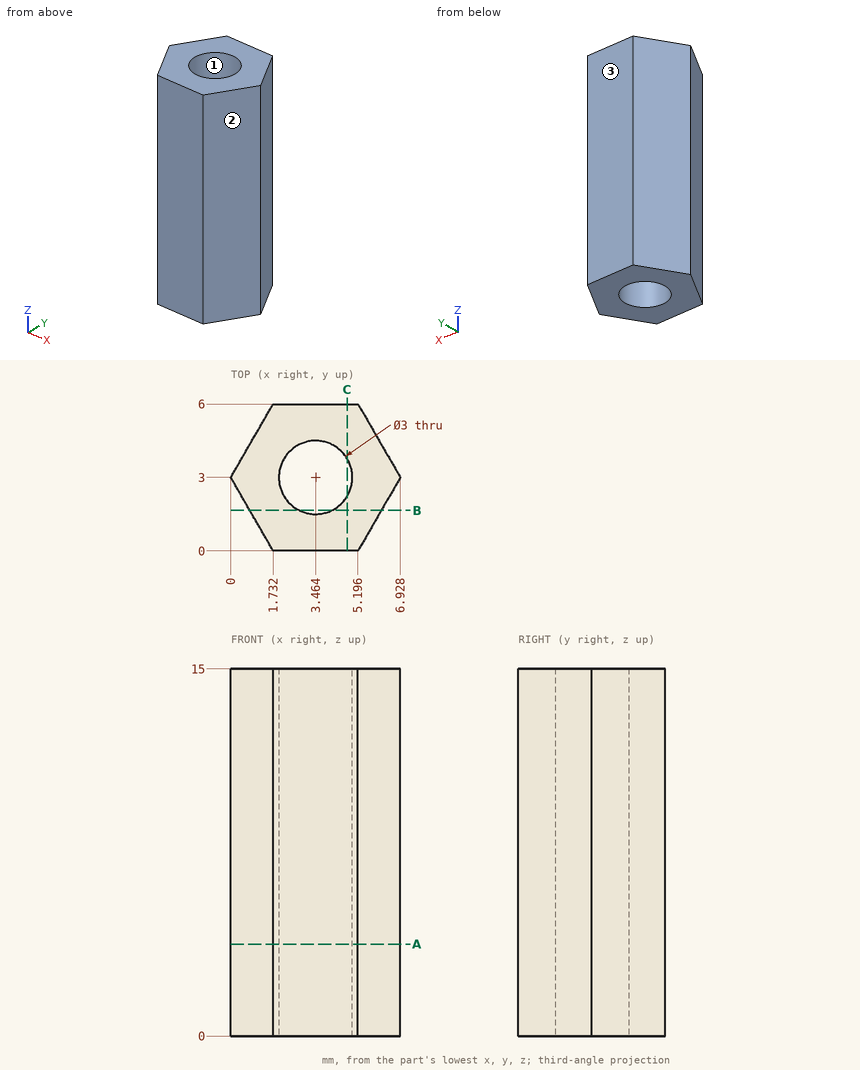
For this review, use the dimensioned drawing (mm, ordinates from the lowest corner) and the shaded views. Coordinates: 2 decimals unless noted, no trailing zeros. Order: outer loops, then holes, each group sorted by start corner. A loop starts at its lowest first (then second) coordinate and runs counter-clockwise, first axis right, second up. Notation, with made-up numbers: (-3, 63) -> (41, 63) arc R19 ccw to (41, 70) -> close; hole circle Ø1 at (52.5, 30.25). An arc over 180 degrees is marked (long way). One line per item, written item: value. Start each with the question number.
Q1. Take a section at A-A, the plane z = 3.75. State the section outline as (x, y) points.
Q2. Mouldability with a two-part tool opening along Y and no side actions: class the marked faces 1, 2 and 3 as pulls with the +Y half, pulls with the -Y half, needs draft (parallel to the pull), parting line crosses it, or undercut.
Q3. Take a section at C-C, the plane x = 4.75. State the section outline as (y, z) points.
Q4. Take a section at B-B, the plane y = 1.65. State the section outline as (x, z) points.
Q5. Insertion check: pin 1 Ø3 at (y, z) = (2, 5.5) entering from +X. The pin has a flat end and moves straight along its axis. Give the tip position at first contact, or say it passes through.
Q6. For probe 1 along X at (y, z) = (2.25, 13) (1 decimal); probe 2 along Y at (x, z) = (4.25, 13.5); probe 3 along Y at (x, z) = (3.75, 8.25), list the stretches that pass through material, from the lowest coordinate up.
Values follow:
1. outline: (0, 3) -> (1.73, 0) -> (5.2, 0) -> (6.93, 3) -> (5.2, 6) -> (1.73, 6) -> close; hole circle Ø3 at (3.46, 3)
2. face 1: undercut
2. face 2: pulls with the -Y half
2. face 3: pulls with the +Y half
3. outline: (0, 0) -> (2.23, 0) -> (2.23, 15) -> (0, 15) -> close; (3.77, 0) -> (6, 0) -> (6, 15) -> (3.77, 15) -> close
4. outline: (0.78, 0) -> (2.81, 0) -> (2.81, 15) -> (0.78, 15) -> close; (4.12, 0) -> (6.15, 0) -> (6.15, 15) -> (4.12, 15) -> close
5. pin 1: stops at x = 6.93
6. probe 1: x = 0.4 to 2.2, 4.8 to 6.5
6. probe 2: y = 0 to 1.72, 4.28 to 6
6. probe 3: y = 0 to 1.53, 4.47 to 6
